```python
from build123d import *

# Parameters (mm, degrees)
SKETCH1_R           = 4.7
BOSS_EXTRUDE1_DEPTH = 3
SKETCH2_R           = 2.4
BOSS_EXTRUDE2_DEPTH = 20
CUT_EXTRUDE1_DEPTH  = 1.5
CHAMFER1_SIZE       = 0.5


with BuildPart() as part:
    # Sketch1 → Boss-Extrude1 (new body)
    with BuildSketch(Plane(origin=(0, 0, 0), x_dir=(1, 0, 0), z_dir=(0, 1, 0))):
        with Locations(Location((0, 0, 0), (0, 0, 270))):
            Circle(SKETCH1_R)
    extrude(amount=BOSS_EXTRUDE1_DEPTH)

    # Sketch2 → Boss-Extrude2 (add)
    with BuildSketch(Plane(origin=(0, 3, 0), x_dir=(1, 0, 0), z_dir=(0, 1, 0))):
        with Locations(Location((0, 0, 0), (0, 0, 270))):
            Circle(SKETCH2_R)
    extrude(amount=BOSS_EXTRUDE2_DEPTH)

    # Sketch3 → Cut-Revolve1 (revolve, cut)
    with BuildSketch(Plane.XY, mode=Mode.PRIVATE) as cut_revolve1_sk:
        with BuildLine():
            Line((2.35, 0), (4.7, 0))
            Line((4.7, 0), (4.7, 2.85))
            add(Edge.make_bspline(
                [(2.35, 0), (4.432462228, 0.599611143), (4.7, 2.85)],
                knots=[0, 0, 0, 1, 1, 1], degree=2))
        make_face()
    revolve(cut_revolve1_sk.sketch.rotate(Axis((0, 0, 0), (0, 1, 0)), 90), axis=Axis((0, 0, 0), (0, 1, 0)), mode=Mode.SUBTRACT)

    # Sketch4 → Cut-Extrude1 (cut)
    with BuildSketch(Plane.XZ):
        Polygon((0, 1.732050808), (-1.5, 0.866025404), (-1.5, -0.866025404), (0, -1.732050808), (1.5, -0.866025404), (1.5, 0.866025404), align=None)
    extrude(amount=-CUT_EXTRUDE1_DEPTH, mode=Mode.SUBTRACT)

    # Chamfer1
    chamfer1_edges = [part.edges().sort_by_distance(p)[0] for p in [
        (0, 23, -2.4),
    ]]
    chamfer(chamfer1_edges, length=CHAMFER1_SIZE)


solid = part.part
```
Design review of the part built by this model. Coordinates are the model's own, in mm. A direction names the side the tool comes from. Coordinates: 2 decimals unless noted, no trailing zeros. Write each loop counter-clockwise with the first axis right and the second up, starting at its lowest first coordinate (ties: lowest second). Pieces come first, ordered by that corner, then holes. Notation, with made-up numbers: M 32.5,-10 L 36.5,-10 A16 ccw 36.5,10 Z; hole C 33.25,55.25 d5. An arc over 180 degrees is marked long. Answer as a JSON object with one key per item and string values.
Item 1: Wall thickness on probe 1 along X at (y, z) = (13.25, -0.5); probe 2 along Y at (x, z) = (1.75, -0.75); probe 3 along X at (y, z) = (9.5, 0): over which ranges is each line inside the solid? List them lowest first.
Outcome:
{"probe 1": "-2.35 to 2.35", "probe 2": "0 to 23", "probe 3": "-2.4 to 2.4"}
Item 2: Insertion check: pin 1 Ø2 at (y, z) = (13.5, 3.5) entering from -X; pin 2 Ø1.2 at (y, z) = (1, -0.5) entering from +X; pin 3 Ø2.5 at (x, z) = (0.5, 0) entering from -Y; pin 4 Ø5 at (y, z) = (20, 0) entering from -X. Each pin has a flat end and moves straight along its axis. Give the tip position at first contact, or say it passes through.
Outcome:
{"pin 1": "through", "pin 2": "x = 4.33", "pin 3": "y = 0", "pin 4": "x = -2.4"}
Item 3: Add section A-A, the plane y = 7.25. Give the boundary of the cut face in (x, z).
Outcome:
{"outline": "C 0,0 d4.8"}
Item 4: Draft analysis for pull direction X (two halves, no side actions). For faces 1 (the flat face through (0.74, 0.74, -1.305)), 2 (the flat face through (0, 23, 0)), 3 (the cylindrical face through (2.024, 12.614, 1.29)), state which applies: pulls with the +X half, pulls with the -X half, needs draft (parallel to the pull), parting line crosses it, or undercut.
Outcome:
{"face 1": "undercut", "face 2": "needs draft", "face 3": "parting line crosses it"}
Item 5: Machinability: for faces 4 (the flat face through (-2, 0, 0)), 5 (the flat face through (-2, 3, 2)), 6 (the flat face through (0, 1.5, 0)), which of the approach directions +Z, -Z, +X, -X, +Y, -Y give a long, thin tool a straight path to every point of the face, cutting with its end or side? Answer none if there is none.
Outcome:
{"face 4": "+Z, -Z, +X, -X, -Y", "face 5": "+Y", "face 6": "-Y"}
